Verification items for this drawing (mm, ordinates from the low corner). A direction names the side the tool comes from. Coordinates: 2 decimals unless noted, no trailing zeros. Loops run counter-clockwise (first coordinate to the right, second up) from the corner with the lowest first, then second, coordinate; pieces in that order, holes last. Notation, with made-up numbers: (8, -21.5) -> (59, -21.5) arc R14 ccw to (59, -4.5) -> close; hole circle Ø2 at (77, -27). An arc over 180 degrees is marked (long way). Write item = value, one per line.
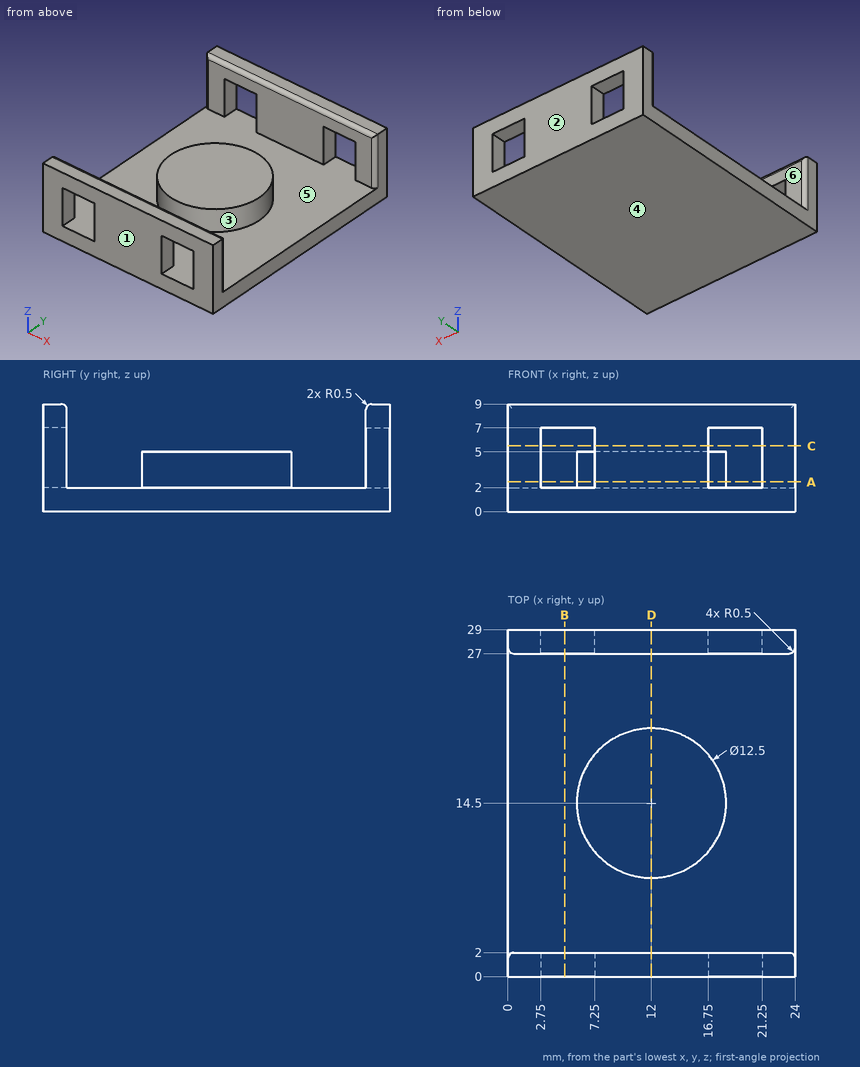
1) Tool access check on the marked faces 4, 5 and 6. Record the directions out of +Z, -Z, +X, -X, +Y, -Y that give a thin tool (end or side, any length) a straight path to the whole face; none if there is none.
Ans:
face_4 = -Z, +X, -X, +Y, -Y
face_5 = none
face_6 = +Z, +X, -X
2) Sectioned sample at C-C, the plane z = 5.5. Record the cut outline in (x, y).
Ans:
outline = (0, 0) -> (2.75, 0) -> (2.75, 2) -> (0.5, 2) arc R0.5 ccw to (0, 1.5) -> close; (0, 27.5) arc R0.5 ccw to (0.5, 27) -> (2.75, 27) -> (2.75, 29) -> (0, 29) -> close; (7.25, 0) -> (16.75, 0) -> (16.75, 2) -> (7.25, 2) -> close; (7.25, 27) -> (16.75, 27) -> (16.75, 29) -> (7.25, 29) -> close; (21.25, 0) -> (24, 0) -> (24, 1.5) arc R0.5 ccw to (23.5, 2) -> (21.25, 2) -> close; (21.25, 27) -> (23.5, 27) arc R0.5 ccw to (24, 27.5) -> (24, 29) -> (21.25, 29) -> close
3) Release check for a two-part mould opening along Y. For the marked faces 1, 2 and 3 record: pulls with the +Y half, pulls with the -Y half, needs draft (parallel to the pull), parting line crosses it, or undercut.
Ans:
face_1 = pulls with the -Y half
face_2 = pulls with the +Y half
face_3 = undercut
4) Sectioned sample at B-B, the plane x = 4.75. Record the cut outline in (y, z).
Ans:
outline = (0, 0) -> (29, 0) -> (29, 2) -> (0, 2) -> close; (0, 7) -> (2, 7) -> (2, 8.5) arc R0.5 ccw to (1.5, 9) -> (0, 9) -> close; (27, 7) -> (29, 7) -> (29, 9) -> (27.5, 9) arc R0.5 ccw to (27, 8.5) -> close
5) Depth check by flat-ended pin: pin 1 Ø1.6 at (x, y) = (18.5, 28) entering from -Z; pin 2 Ø10 at (x, y) = (14.5, 12.5) entering from +Z; pin 3 Ø1.5 at (y, z) = (8.5, 5) entering from -X; pin 4 Ø1.5 at (y, z) = (20, 4.5) entering from -X. Enter the tip coordinate at first touch or a pass-through.
Ans:
pin_1 = 0
pin_2 = 5
pin_3 = 8.61
pin_4 = 7.94
6) Material ranges on line 1 (Y direction, x = 9.5, z = 7.75); line 2 (Y direction, x = 15.75, z = 3); line 3 (Z direction, x = 21, y = 21.25), recorded low to high.
Ans:
line_1 = 0 to 2, 27 to 29
line_2 = 0 to 2, 9.5 to 19.5, 27 to 29
line_3 = 0 to 2
7) Sectioned sample at A-A, the plane z = 2.5. Count the separate pieces of the cut face and the enclosed holes in it, plus the area to 3 significant figures.
Ans:
separate_pieces = 7
enclosed_holes = 0
area = 183 mm2
8) Sectioned sample at D-D, the plane x = 12. Record the cut outline in (y, z), plus the area to 3 significant figures.
Ans:
outline = (0, 0) -> (29, 0) -> (29, 9) -> (27.5, 9) arc R0.5 ccw to (27, 8.5) -> (27, 2) -> (20.75, 2) -> (20.75, 5) -> (8.25, 5) -> (8.25, 2) -> (2, 2) -> (2, 8.5) arc R0.5 ccw to (1.5, 9) -> (0, 9) -> close
area = 123 mm2
